```python
from build123d import *

# Parameters (mm, degrees)
SKETCH1_W           = 21.336
SKETCH1_H           = 16.51
SKETCH1_R           = 1.524
BOSS_EXTRUDE1_DEPTH = 2.7
SKETCH2_OUTSIDE_W   = 28.758
SKETCH2_OUTSIDE_H   = 23.932
SKETCH2_OUTSIDE_W_2 = 4.064
SKETCH2_OUTSIDE_H_2 = 4.064
CUT_EXTRUDE1_DEPTH  = 1.6002


with BuildPart() as part:
    # Sketch1 → Boss-Extrude1 (new body)
    with BuildSketch(Plane.XY):
        with Locations((10.668, 8.255)):
            Rectangle(SKETCH1_W, SKETCH1_H)
        with Locations((2.168, 2.168)):
            Circle(SKETCH1_R, mode=Mode.SUBTRACT)
        with Locations((19.168, 2.168)):
            Circle(SKETCH1_R, mode=Mode.SUBTRACT)
    extrude(amount=BOSS_EXTRUDE1_DEPTH)

    # Sketch2 outside → Cut-Extrude1 (cut)
    with BuildSketch(Plane.XY.offset(2.7)):
        with Locations((10.668, 8.255)):
            Rectangle(SKETCH2_OUTSIDE_W, SKETCH2_OUTSIDE_H)
        with Locations((10.668, 6.7564)):
            Rectangle(SKETCH2_OUTSIDE_W_2, SKETCH2_OUTSIDE_H_2, mode=Mode.SUBTRACT)
    extrude(amount=-CUT_EXTRUDE1_DEPTH, mode=Mode.SUBTRACT)


solid = part.part
```
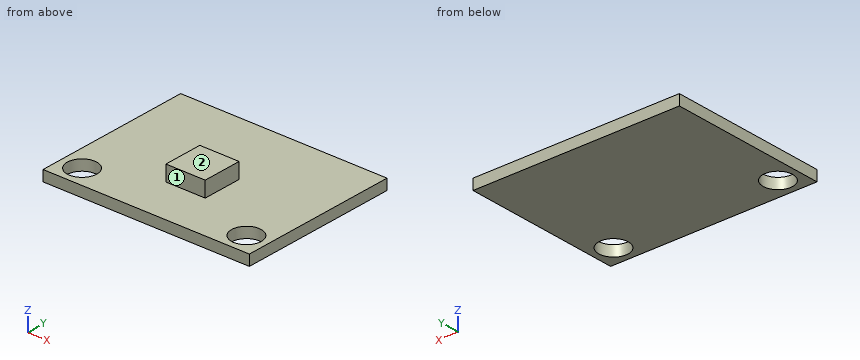
Can you work these out from the model? Positions are in its coordinate system, mm. Face numbers are marked on the shaded views. A direction names the side the tool comes from. Give positions to 0.01 mm unless a question says otherwise; leave off trailing zeros. Order: outer loops, then holes, each group sorted by start corner. A loop starts at its lowest first (then second) coordinate and runs counter-clockwise, first axis right, second up. Notation, with made-up numbers: M 42.25,45.25 L 53.25,45.25 A14 cw 53.25,63.25 Z; hole C -36.5,-29 d2. An arc over 180 degrees is marked long. Write item = value, one per line. Start each with the question number.
Q1. Suppose I cut it at C-C (y = 2.5). Write out the boundary of the cut face in (x, z), plus the area to 3 significant figures.
Q2. For the marked faces 1 and 2, which set-ups out of +Z, -Z, +X, -X, +Y, -Y let a thin tool reach every point of the face, with its end or its side?
Q3. Suppose I cut it at B-B (y = 7.25). Write out the boundary of the cut face in (x, z).
Q4. I need wall thicknesses on probe 1 along X at (y, z) = (1, 0.75); probe 2 along Z at (x, y) = (15.25, 9.75); probe 3 along X at (y, z) = (8.25, 2.5). Which ranges of each line are inside material? Lowest first, please. Write a range as [from, to].
Q5. Suppose I cut it at A-A (x = 11). Write out the boundary of the cut face in (y, z).
Q6. Will these pins go through, and if not, where does the flat tip stop? pin 1 Ø1.5 at (x, y) = (2, 9.5) entering from +Z; pin 2 Ø1.8 at (x, y) = (19.168, 2.168) entering from +Z; pin 3 Ø0.5 at (x, z) = (10, 2) entering from +Y; pin 4 Ø0.5 at (y, z) = (6.5, 2.5) entering from +X.
Q7. Suppose I cut it at D-D (z = 1.6). Write out the boundary of the cut face in (x, y), plus the area to 3 significant figures.
Check result:
q1.outline = M 0,0 L 0.68,0 L 0.68,1.1 L 0,1.1 Z; M 3.66,0 L 17.68,0 L 17.68,1.1 L 3.66,1.1 Z; M 20.66,0 L 21.34,0 L 21.34,1.1 L 20.66,1.1 Z
q1.area = 16.9 mm2
q2.face_1 = +Z, +X, -X, -Y
q2.face_2 = +Z, +X, -X, +Y, -Y
q3.outline = M 0,0 L 21.34,0 L 21.34,1.1 L 12.7,1.1 L 12.7,2.7 L 8.64,2.7 L 8.64,1.1 L 0,1.1 Z
q4.probe_1 = [0, 1.19], [3.15, 18.19], [20.15, 21.34]
q4.probe_2 = [0, 1.1]
q4.probe_3 = [8.64, 12.7]
q5.outline = M 0,0 L 16.51,0 L 16.51,1.1 L 8.79,1.1 L 8.79,2.7 L 4.72,2.7 L 4.72,1.1 L 0,1.1 Z
q6.pin_1 = 1.1
q6.pin_2 = through
q6.pin_3 = 8.79
q6.pin_4 = 12.7
q7.outline = M 8.64,4.72 L 12.7,4.72 L 12.7,8.79 L 8.64,8.79 Z
q7.area = 16.5 mm2
